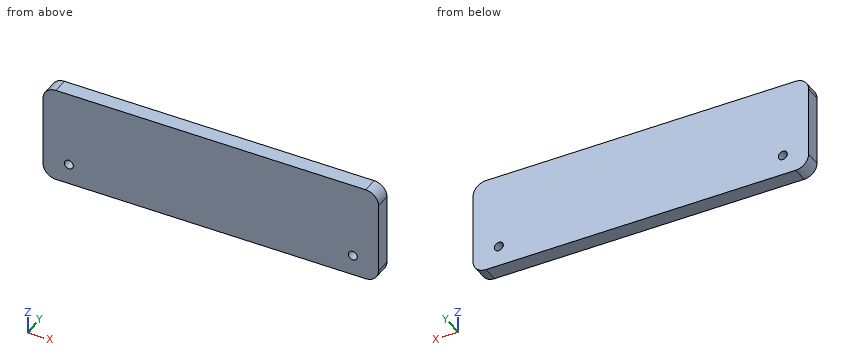
```python
from build123d import *

# Parameters (mm, degrees)
SKETCH1_W           = 130
SKETCH1_H           = 37.5
BOSS_EXTRUDE1_DEPTH = 6
FILLET1_R           = 5
SKETCH2_R           = 1.75
CUT_EXTRUDE1_DEPTH  = 6


with BuildPart() as part:
    # Sketch1 → Boss-Extrude1 (new body)
    with BuildSketch(Plane(origin=(0, 0, 0), x_dir=(1, 0, 0), z_dir=(0, 1, 0))):
        with Locations((65, 18.75)):
            Rectangle(SKETCH1_W, SKETCH1_H)
    extrude(amount=BOSS_EXTRUDE1_DEPTH)

    # Fillet1
    fillet1_edges = [part.edges().sort_by_distance(p)[0] for p in [
        (0, 3, -37.5),
        (130, 3, -37.5),
        (130, 3, 0),
        (0, 3, 0),
    ]]
    fillet(fillet1_edges, radius=FILLET1_R)

    # Sketch2 → Cut-Extrude1 (cut)
    with BuildSketch(Plane(origin=(0, 6, 0), x_dir=(1, 0, 0), z_dir=(0, 1, 0))):
        with Locations((10, 29.5)):
            Circle(SKETCH2_R)
        with Locations((120, 29.5)):
            Circle(SKETCH2_R)
    extrude(amount=-CUT_EXTRUDE1_DEPTH, mode=Mode.SUBTRACT)


solid = part.part
```
Here's how the part is built. I have some questions about the finished solid (model axes, mm). Coordinates: 2 decimals unless noted, no trailing zeros. Order: outer loops, then holes, each group sorted by start corner. A loop starts at its lowest first (then second) coordinate and runs counter-clockwise, first axis right, second up. Notation, with made-up numbers: (-26.5, -29.5) - (12.5, -29.5) arc R30 cw to (12.5, 4.5) - close; hole circle Ø1 at (14, 68.5). An arc over 180 degrees is marked (long way). One line per question, with ' | ' between items. Start each with the question number.
1. I'm going to push a flat-ended pin straight in: pin 1 Ø3 at (x, z) = (120, -29.5) entering from +Y. Where does the tip first touch, or does it pass through?
2. If we section it at B-B (x = 10): Write out the boundary of the cut face in (y, z).
3. Please list where these lines run through material, in increasing order: line 1 along X through (y, z) = (3.4, -29.5); line 2 along Z through (x, y) = (120, 3.35); line 3 along Z through (x, y) = (121, 0.5). Write a range as [from, to].
4. If we section it at A-A (z = -29.5): Write out the boundary of the cut face in (x, y).
Model answer:
1) pin 1: passes through
2) outline: (0, -37.5) - (6, -37.5) - (6, -31.25) - (0, -31.25) - close; (0, -27.75) - (6, -27.75) - (6, 0) - (0, 0) - close
3) line 1: x = [0, 8.25], [11.75, 118.25], [121.75, 130] | line 2: z = [-37.5, -31.25], [-27.75, 0] | line 3: z = [-37.5, -30.94], [-28.06, 0]
4) outline: (0, 0) - (8.25, 0) - (8.25, 6) - (0, 6) - close; (11.75, 0) - (118.25, 0) - (118.25, 6) - (11.75, 6) - close; (121.75, 0) - (130, 0) - (130, 6) - (121.75, 6) - close
